from build123d import *
from OCP.BRepFilletAPI import BRepFilletAPI_MakeChamfer

# Parameters (mm, degrees)
EXTRUSION1_DEPTH        = 4.5
EXTRUSION2_DEPTH        = 1.48
EXTRUSION2_DEPTH_BACK   = 6.5
ESQUISSE3_R             = 0.625
CONG_1_R                = 0.2
CHANFREIN1_SIZE         = 0.2
CHANFREIN1_SIZE2        = 0.238350719
ESQUISSE4_W             = 3.88
ESQUISSE4_H             = 1.2
ENL_V_MAT_EXTRU_1_DEPTH = 1.5
EXTRUSION3_DEPTH        = 0.4
ESQUISSE8_W             = 0.420106654
ESQUISSE8_H             = 8.687057787
EXTRUSION4_DEPTH        = 5
ESQUISSE9_W             = 0.424689677
ESQUISSE9_H             = 1.25
EXTRUSION5_DEPTH        = 2.5
CONG_3_R                = 0.5
CONG_4_R                = 0.5
ESQUISSE11_R            = 3.45
EXTRUSION6_DEPTH        = 1.36
ESQUISSE12_R            = 3.1
ENL_V_MAT_EXTRU_2_DEPTH = 4
ESQUISSE13_R            = 3.05
EXTRUSION7_DEPTH        = 11
ESQUISSE14_W            = 7.136387573
ESQUISSE14_H            = 2.568018255
ENL_V_MAT_EXTRU_7_DEPTH = 6
CHANFREIN2_SIZE         = 0.3
CHANFREIN2_SIZE2        = 0.357526078
ESQUISSE15_W            = 1.5
ESQUISSE15_H            = 0.42
EXTRUSION8_DEPTH        = 0.65
ESQUISSE16_W            = 1.5
ESQUISSE16_H            = 0.42
EXTRUSION9_DEPTH        = 3
ESQUISSE17_W            = 0.8
ESQUISSE17_H            = 0.42
EXTRUSION10_DEPTH       = 3.5
CONG_5_R                = 0.4
ESQUISSE18_W            = 0.420106654
ESQUISSE18_H            = 3
EXTRUSION11_DEPTH       = 1.5
ESQUISSE19_W            = 0.420106654
ESQUISSE19_H            = 2
EXTRUSION12_DEPTH       = 3.8
CONG_6_R                = 1
CONG_3_OF_SYM_TRIE1_R   = 0.5
CONG_4_OF_SYM_TRIE1_R   = 0.5
CONG_6_OF_SYM_TRIE1_R   = 1


with BuildPart() as part:
    # Esquisse2 → Extrusion1 (new body)
    with BuildSketch(Plane.XY):
        with BuildLine():
            Line((-3.375, 5.95), (3.375, 5.95))
            ThreePointArc((3.375, 5.95), (4.082106781, 5.657106781), (4.375, 4.95))
            Line((4.375, 4.95), (4.375, -4.95))
            ThreePointArc((4.375, -4.95), (4.082106781, -5.657106781), (3.375, -5.95))
            Line((3.375, -5.95), (-3.375, -5.95))
            ThreePointArc((-3.375, -5.95), (-4.082106781, -5.657106781), (-4.375, -4.95))
            Line((-4.375, -4.95), (-4.375, 4.95))
            ThreePointArc((-4.375, 4.95), (-4.082106781, 5.657106781), (-3.375, 5.95))
        make_face()
    extrude(amount=EXTRUSION1_DEPTH)

    # Esquisse3 → Extrusion2 (add, two sides: drawn at the far end of the back side and taken through both)
    with BuildSketch(Plane.XY.offset(4.5).offset(-EXTRUSION2_DEPTH_BACK)):
        with Locations((-2.75, 4.725)):
            Circle(ESQUISSE3_R)
        with Locations((2.75, 4.725)):
            Circle(ESQUISSE3_R)
        with Locations((2.75, -3.695)):
            Circle(ESQUISSE3_R)
        with Locations((-2.75, -3.695)):
            Circle(ESQUISSE3_R)
    extrude(amount=EXTRUSION2_DEPTH + EXTRUSION2_DEPTH_BACK)

    # Congé1
    cong_1_edges = [part.edges().sort_by_distance(p)[0] for p in [
        (-3.375, 4.725, 5.98),
        (2.125, 4.725, 5.98),
        (2.125, -3.695, 5.98),
        (-3.375, -3.695, 5.98),
    ]]
    fillet(cong_1_edges, radius=CONG_1_R)

    # Chanfrein1: one chamfer whose edges measure the first distance from different faces: ONE call of the kernel's chamfer builder (chamfer() names one face for all edges)
    chanfrein1_edges_1 = [part.edges().sort_by_distance(p)[0] for p in [
        (-3.375, 4.725, -2),
    ]]
    chanfrein1_side_1 = [part.faces().sort_by_distance(p)[0] for p in [
        (-2.75, 4.725, -2),
    ]]
    chanfrein1_edges_2 = [part.edges().sort_by_distance(p)[0] for p in [
        (2.125, 4.725, -2),
    ]]
    chanfrein1_side_2 = [part.faces().sort_by_distance(p)[0] for p in [
        (2.75, 4.725, -2),
    ]]
    chanfrein1_edges_3 = [part.edges().sort_by_distance(p)[0] for p in [
        (2.125, -3.695, -2),
    ]]
    chanfrein1_side_3 = [part.faces().sort_by_distance(p)[0] for p in [
        (2.75, -3.695, -2),
    ]]
    chanfrein1_edges_4 = [part.edges().sort_by_distance(p)[0] for p in [
        (-3.375, -3.695, -2),
    ]]
    chanfrein1_side_4 = [part.faces().sort_by_distance(p)[0] for p in [
        (-2.75, -3.695, -2),
    ]]
    chanfrein1 = BRepFilletAPI_MakeChamfer(part.part.solid().wrapped)
    for e in chanfrein1_edges_1:
        chanfrein1.Add(CHANFREIN1_SIZE, CHANFREIN1_SIZE2, e.wrapped, chanfrein1_side_1[0].wrapped)  # the first distance lies on this face
    for e in chanfrein1_edges_2:
        chanfrein1.Add(CHANFREIN1_SIZE, CHANFREIN1_SIZE2, e.wrapped, chanfrein1_side_2[0].wrapped)  # the first distance lies on this face
    for e in chanfrein1_edges_3:
        chanfrein1.Add(CHANFREIN1_SIZE, CHANFREIN1_SIZE2, e.wrapped, chanfrein1_side_3[0].wrapped)  # the first distance lies on this face
    for e in chanfrein1_edges_4:
        chanfrein1.Add(CHANFREIN1_SIZE, CHANFREIN1_SIZE2, e.wrapped, chanfrein1_side_4[0].wrapped)  # the first distance lies on this face
    add(Compound.cast(chanfrein1.Shape()), mode=Mode.REPLACE)

    # Esquisse4 → Enlèv. mat.-Extru.1 (cut)
    with BuildSketch(Plane.XY.offset(4.5)):
        with Locations((0, -5.35)):
            Rectangle(ESQUISSE4_W, ESQUISSE4_H)
    extrude(amount=-ENL_V_MAT_EXTRU_1_DEPTH, mode=Mode.SUBTRACT)

    # Esquisse5 → Extrusion3 (add)
    with BuildSketch(Plane.XY.offset(4.5)):
        with BuildLine():
            Line((-3.375865226, 5.937057787), (0, 5.937057787))
            Line((0, 5.937057787), (0, -4.775009367))
            Line((0, -4.775009367), (-3.376178009, -4.775009367))
            ThreePointArc((-3.376178009, -4.775009367), (-4.092072333, -4.473218015), (-4.375865226, -3.75))
            Line((-4.375865226, -3.75), (-4.875865226, -3.75))
            Line((-4.875865226, -3.75), (-4.875865226, 4.937057787))
            Line((-4.875865226, 4.937057787), (-4.375865226, 4.937057787))
            ThreePointArc((-4.375865226, 4.937057787), (-4.082972007, 5.644164569), (-3.375865226, 5.937057787))
        make_face()
    extrusion3 = extrude(amount=EXTRUSION3_DEPTH)

    # Esquisse8 → Extrusion4 (add)
    with BuildSketch(Plane(origin=(0, 0, 4.5), x_dir=(-1, 0, 0), z_dir=(0, 0, -1))):
        with Locations((4.665811899, 0.593528894)):
            Rectangle(ESQUISSE8_W, ESQUISSE8_H)
    extrusion4 = extrude(amount=EXTRUSION4_DEPTH)

    # Esquisse9 → Extrusion5 (add)
    with BuildSketch(Plane(origin=(-4.455758572, 0, 0), x_dir=(0, 0, -1), z_dir=(1, 0, 0))):
        with Locations((0.283831247, -2.075)):
            Rectangle(ESQUISSE9_W, ESQUISSE9_H)
        with Locations((0.284099775, 3.325)):
            Rectangle(ESQUISSE9_W, ESQUISSE9_H)
    extrusion5 = extrude(amount=EXTRUSION5_DEPTH)

    # Congé3
    cong_3_edges = [part.edges().sort_by_distance(p)[0] for p in [
        (-1.955758572, -1.45, -0.283831246),
        (-1.955758572, -2.7, -0.283831246),
    ]]
    fillet(cong_3_edges, radius=CONG_3_R)

    # Congé4
    cong_4_edges = [part.edges().sort_by_distance(p)[0] for p in [
        (-1.955758572, 3.95, -0.284099776),
        (-1.955758572, 2.7, -0.284099776),
    ]]
    fillet(cong_4_edges, radius=CONG_4_R)

    # Esquisse11 → Extrusion6 (add)
    with BuildSketch(Plane.XY.offset(4.9)):
        with Locations(Location((0, 0, 0), (0, 0, 270))):
            Circle(ESQUISSE11_R)
    extrude(amount=EXTRUSION6_DEPTH)

    # Esquisse12 → Enlèv. mat.-Extru.2 (cut)
    with BuildSketch(Plane.XY.offset(6.26)):
        Circle(ESQUISSE12_R)
    extrude(amount=-ENL_V_MAT_EXTRU_2_DEPTH, mode=Mode.SUBTRACT)

    # Esquisse13 → Extrusion7 (add)
    with BuildSketch(Plane.XY.offset(2.26)):
        Circle(ESQUISSE13_R)
    extrude(amount=EXTRUSION7_DEPTH)

    # Esquisse14 → Enlèv. mat.-Extru.7 (cut)
    with BuildSketch(Plane.XY.offset(13.26)):
        with Locations((0.012650659, 2.216605231)):
            Rectangle(ESQUISSE14_W, ESQUISSE14_H)
    extrude(amount=-ENL_V_MAT_EXTRU_7_DEPTH, mode=Mode.SUBTRACT)

    # Chanfrein2
    chanfrein2_edges = [part.edges().sort_by_distance(p)[0] for p in [
        (-0.471983632, -3.013259274, 13.26),
        (0, 0.932596103, 13.26),
    ]]
    chanfrein2_side = [part.faces().sort_by_distance(p)[0] for p in [
        (0, -0.80773857, 13.26),
    ]]
    chamfer(chanfrein2_edges, length=CHANFREIN2_SIZE, length2=CHANFREIN2_SIZE2, reference=chanfrein2_side[0])

    # Esquisse15 → Extrusion8 (add)
    with BuildSketch(Plane.XZ.offset(5.95)):
        with Locations((0, 1.69)):
            Rectangle(ESQUISSE15_W, ESQUISSE15_H)
        with Locations((2.5, 1.69)):
            Rectangle(ESQUISSE15_W, ESQUISSE15_H)
        with Locations((-2.5, 1.69)):
            Rectangle(ESQUISSE15_W, ESQUISSE15_H)
    extrude(amount=EXTRUSION8_DEPTH)

    # Esquisse16 → Extrusion9 (add)
    with BuildSketch(Plane(origin=(0, 0, 1.48), x_dir=(-1, 0, 0), z_dir=(0, 0, -1))):
        with Locations((2.5, -6.39)):
            Rectangle(ESQUISSE16_W, ESQUISSE16_H)
        with Locations((0, -6.39)):
            Rectangle(ESQUISSE16_W, ESQUISSE16_H)
        with Locations((-2.5, -6.39)):
            Rectangle(ESQUISSE16_W, ESQUISSE16_H)
    extrude(amount=EXTRUSION9_DEPTH)

    # Esquisse17 → Extrusion10 (add)
    with BuildSketch(Plane(origin=(0, 0, -1.52), x_dir=(-1, 0, 0), z_dir=(0, 0, -1))):
        with Locations((2.5, -6.39)):
            Rectangle(ESQUISSE17_W, ESQUISSE17_H)
        with Locations((0, -6.39)):
            Rectangle(ESQUISSE17_W, ESQUISSE17_H)
        with Locations((-2.5, -6.39)):
            Rectangle(ESQUISSE17_W, ESQUISSE17_H)
    extrude(amount=EXTRUSION10_DEPTH)

    # Congé5
    cong_5_edges = [part.edges().sort_by_distance(p)[0] for p in [
        (2.9, -6.39, -5.02),
        (-2.1, -6.39, -5.02),
        (0.4, -6.39, -5.02),
        (-2.9, -6.39, -5.02),
        (-0.4, -6.39, -5.02),
        (2.1, -6.39, -5.02),
    ]]
    fillet(cong_5_edges, radius=CONG_5_R - 0.0001)  # a hair under: the kernel refuses the full size

    # Esquisse18 → Extrusion11 (add)
    with BuildSketch(Plane(origin=(0, 0, -0.5), x_dir=(-1, 0, 0), z_dir=(0, 0, -1))):
        with Locations((4.665811899, 0.625)):
            Rectangle(ESQUISSE18_W, ESQUISSE18_H)
    extrusion11 = extrude(amount=EXTRUSION11_DEPTH)

    # Esquisse19 → Extrusion12 (add)
    with BuildSketch(Plane(origin=(0, 0, -2), x_dir=(-1, 0, 0), z_dir=(0, 0, -1))):
        with Locations((4.665811899, 0.625)):
            Rectangle(ESQUISSE19_W, ESQUISSE19_H)
    extrusion12 = extrude(amount=EXTRUSION12_DEPTH)

    # Congé6
    cong_6_edges = [part.edges().sort_by_distance(p)[0] for p in [
        (-4.665811899, -0.375, -5.8),
        (-4.665811899, 1.625, -5.8),
    ]]
    fillet(cong_6_edges, radius=CONG_6_R - 0.0001)  # a hair under: the kernel refuses the full size

    # Symétrie1: Extrusion3, Extrusion4, Extrusion5, Extrusion11, Extrusion12 across Right Plane
    add(extrusion3.mirror(Plane(origin=(0, 0, 0), x_dir=(0, 0, -1), z_dir=(1, 0, 0))))
    add(extrusion4.mirror(Plane(origin=(0, 0, 0), x_dir=(0, 0, -1), z_dir=(1, 0, 0))))
    add(extrusion5.mirror(Plane(origin=(0, 0, 0), x_dir=(0, 0, -1), z_dir=(1, 0, 0))))
    add(extrusion11.mirror(Plane(origin=(0, 0, 0), x_dir=(0, 0, -1), z_dir=(1, 0, 0))))
    add(extrusion12.mirror(Plane(origin=(0, 0, 0), x_dir=(0, 0, -1), z_dir=(1, 0, 0))))

    # Congé3 of Symétrie1
    cong_3_of_sym_trie1_edges = [part.edges().sort_by_distance(p)[0] for p in [
        (1.955758572, -1.45, -0.283831246),
        (1.955758572, -2.7, -0.283831246),
    ]]
    fillet(cong_3_of_sym_trie1_edges, radius=CONG_3_OF_SYM_TRIE1_R)

    # Congé4 of Symétrie1
    cong_4_of_sym_trie1_edges = [part.edges().sort_by_distance(p)[0] for p in [
        (1.955758572, 3.95, -0.284099776),
        (1.955758572, 2.7, -0.284099776),
    ]]
    fillet(cong_4_of_sym_trie1_edges, radius=CONG_4_OF_SYM_TRIE1_R)

    # Congé6 of Symétrie1
    cong_6_of_sym_trie1_edges = [part.edges().sort_by_distance(p)[0] for p in [
        (4.665811899, -0.375, -5.8),
        (4.665811899, 1.625, -5.8),
    ]]
    fillet(cong_6_of_sym_trie1_edges, radius=CONG_6_OF_SYM_TRIE1_R - 0.0001)  # a hair under: the kernel refuses the full size


solid = part.part
Can you work these out from the model? Positions are in its coordinate system, mm. A direction names the side the tool comes from. Round coordinates to 2 decimals unless told otherwise and drop trailing zeros. Write each loop counter-clockwise with the first axis right and the second up, starting at its lowest first coordinate (ties: lowest second). Pieces come first, ordered by that corner, then holes. Notation, with made-up numbers: (53, 13) - (104, 13) arc R17 ccw to (104, 35) - close; hole circle Ø11 at (34.5, -33). An arc over 180 degrees is marked (long way). Write each question's results on one line, items separated by ' | '. Start each with the question number.
1) Suppose I cut it at A-A (z = 3.75). List the corners of the cut face in (x, y) for me (3 decimals).
2) Please list where these lines run through material, in increasing order: line 1 (Y direction, x = -2.75, z = -1.25); line 2 (Z direction, x = -3, y = -4); line 3 (Y direction, x = -1.75, z = 7).
3) Suppose I cut it at B-B (z = -1.25). Give the number of separate pieces and of enclosed holes in the cut face, and give its area (3 significant figures).
4) Which directions (+Z, -Z, +X, -X, +Y, -Y) give clear straight access to the entire face, cutting with the end or side of a thin tool? Please do faces 4 (the flat face through (-2.8, 4.7, 5.98)), 5 (the cylindrical face through (2.29, 5.15, 5.33)), 6 (the cylindrical face through (-3.374, 4.752, -0.893)), 7 (the flat face through (-2.8, -3.7, -2)).
5) We'd pull the mould along Y, two halves only. Please class faces 1 (the flat face through (0, -1, 13.26)), 2 (the cylindrical face through (2.669, -3.075, 5.334)), 3 (the cylindrical face through (-4.074, -5.665, 2.218)): released by +Y, released by -Y, zero draft, split by the parting line, or undercut.
6) Suppose I cut it at C-C (z = 11). List the corners of the cut face in (x, y) for me.
7) For pin 1 Ø0.6 at (x, y) = (-3, -2) entering from -Z; pin 2 Ø0.5 at (x, z) = (-4.5, -1) entering from -Y (3 decimals); pin 3 Ø4 at (x, y) = (3.5, -3.5) entering from -Z, each with a flat end and sliding along its axis, tell me the tip position at first contact or that it passes through.
Here are the results:
1) outline: (-4.876, -3.75) - (-4.456, -3.75) - (-4.456, 4.937) - (-4.876, 4.937) - close; (-4.375, -4.95) arc R1 ccw to (-3.375, -5.95) - (-1.94, -5.95) - (-1.94, -4.75) - (1.94, -4.75) - (1.94, -5.95) - (3.375, -5.95) arc R1 ccw to (4.375, -4.95) - (4.375, 4.95) arc R1 ccw to (3.375, 5.95) - (-3.375, 5.95) arc R1 ccw to (-4.375, 4.95) - close; circle Ø6.1 at (0, 0); (4.456, -3.75) - (4.876, -3.75) - (4.876, 4.937) - (4.456, 4.937) - close; hole circle Ø6.2 at (0, 0)
2) line 1: y = -6.6 to -6.18, -4.32 to -3.07, 4.1 to 5.35 | line 2: z = -2 to 5.98 | line 3: y = -2.5 to 2.5
3) separate pieces: 9 | enclosed holes: 0 | area: 9.32 mm2
4) face 4: +Z, +X, -X, +Y | face 5: +Z | face 6: -Z | face 7: -Z, +X, -X, +Y
5) face 1: zero draft | face 2: undercut | face 3: released by -Y
6) outline: (-2.9, 0.93) arc R3.05 ccw (long way) to (2.9, 0.93) - close
7) pin 1: stops at z = -0.5 | pin 2: stops at y = -0.875 | pin 3: stops at z = -2
